Check sheet for the modelled part. Datum: model origin and axes. Units: mm. A direction names the side the tool comes from. Coordinates: 2 decimals unless noted, no trailing zeros. Loops run counter-clockwise (first coordinate to the right, second up) from the corner with the lowest first, then second, coordinate; pieces in that order, holes last. Notation, with made-up numbers: M -19,27.5 L 14,27.5 A21 ccw 14,34.5 Z; hole C 85.5,-26 d1. An arc over 180 degrees is marked long. Answer in a Markdown table with one row per item. Add a question column.
```python
from build123d import *

# Parameters (mm, degrees)
SKETCH_1_W          = 80
SKETCH_1_H          = 28
SKETCH_1_R          = 4.25
SKETCH_1_R_2        = 2
EXTRUDE_1_DEPTH     = 3
FILLET_2_RADIUS     = 14
FILLET_2_LENGTH     = 3
EXTRUDE_3_DEPTH     = 3
SKETCH_5_W          = 18.5
SKETCH_5_H          = 18.5
EXTRUDE_4_DEPTH     = 3
FILLET_3_R          = 18.5
EXTRUDE_5_DEPTH     = 3
CUT_EXTRUDE_1_REACH = 70.323
SKETCH_10_R         = 1.75


with BuildPart() as part:
    # 草图1 → 凸台-拉伸1 (new body)
    with BuildSketch(Plane(origin=(0, 0, 0), x_dir=(1, 0, 0), z_dir=(0, 1, 0))):
        Rectangle(SKETCH_1_W, SKETCH_1_H)
        with Locations(Location((25, 0, 0), (0, 0, 270))):
            Circle(SKETCH_1_R, mode=Mode.SUBTRACT)
        with Locations(Location((-25, 0, 0), (0, 0, 270))):
            Circle(SKETCH_1_R_2, mode=Mode.SUBTRACT)
    extrude(amount=EXTRUDE_1_DEPTH)

    # 圆角2: full round fillet: the end face becomes a half cylinder, R = half its width
    fillet_2_face = Plane((40, 1.5, 0), x_dir=(0, -1, 0), z_dir=(1, 0, 0))  # on the end face: x along it, z out of the body
    fillet_2_slab = fillet_2_face.offset(-FILLET_2_RADIUS / 2) * Box(FILLET_2_LENGTH, 2 * FILLET_2_RADIUS, FILLET_2_RADIUS, mode=Mode.PRIVATE)  # the body's end, R deep
    fillet_2_round = Plane((26, 1.5, 0), x_dir=(1, 0, 0), z_dir=(0, -1, 0)) * Cylinder(FILLET_2_RADIUS, FILLET_2_LENGTH, mode=Mode.PRIVATE)  # its axis R under the face
    add(fillet_2_slab - fillet_2_round, mode=Mode.SUBTRACT)

    # 草图4 → 凸台-拉伸3 (add)
    with BuildSketch(Plane.XZ):
        with BuildLine():
            Line((-40, 14), (-40, -14))
            ThreePointArc((-40, -14), (-54, 0), (-40, 14))
        make_face()
    extrude(amount=-EXTRUDE_3_DEPTH)

    # 草图5 → 凸台-拉伸4 (add)
    with BuildSketch(Plane(origin=(0, 0, 0), x_dir=(-1, 0, 0), z_dir=(0, -1, 0))):
        with Locations((12.25, -23.25)):
            Rectangle(SKETCH_5_W, SKETCH_5_H)
    extrude(amount=-EXTRUDE_4_DEPTH)

    # 圆角3
    fillet_3_edges = [part.edges().sort_by_distance(p)[0] for p in [
        (-21.5, 1.5, 14),
        (-3, 1.5, 14),
    ]]
    fillet(fillet_3_edges, radius=FILLET_3_R - 0.0001)  # a hair under: the kernel refuses the full size

    # 草图6 → 凸台-拉伸5 (add)
    with BuildSketch(Plane.XZ):
        with BuildLine():
            Line((-21.5, 32.5), (-3, 32.5))
            ThreePointArc((-3, 32.5), (-12.25, 41.75), (-21.5, 32.5))
        make_face()
    extrude(amount=-EXTRUDE_5_DEPTH)

    # 草图10 → 切除-拉伸1 (cut, up to next)
    with BuildSketch(Plane.XZ, mode=Mode.PRIVATE) as cut_extrude_1_sk1:
        with Locations(Location((-12.25, 37.5, 0), (0, 0, 270))):
            Circle(SKETCH_10_R)
    cut_extrude_1_tool1 = extrude(cut_extrude_1_sk1.sketch, amount=-CUT_EXTRUDE_1_REACH, mode=Mode.PRIVATE) & part.part
    # 草图10 → 切除-拉伸1 (cut, up to next)
    with BuildSketch(Plane.XZ, mode=Mode.PRIVATE) as cut_extrude_1_sk2:
        with Locations(Location((-7.919872981, 30, 0), (0, 0, 270))):
            Circle(SKETCH_10_R)
    cut_extrude_1_tool2 = extrude(cut_extrude_1_sk2.sketch, amount=-CUT_EXTRUDE_1_REACH, mode=Mode.PRIVATE) & part.part
    # 草图10 → 切除-拉伸1 (cut, up to next)
    with BuildSketch(Plane.XZ, mode=Mode.PRIVATE) as cut_extrude_1_sk3:
        with Locations(Location((-16.580127019, 30, 0), (0, 0, 270))):
            Circle(SKETCH_10_R)
    cut_extrude_1_tool3 = extrude(cut_extrude_1_sk3.sketch, amount=-CUT_EXTRUDE_1_REACH, mode=Mode.PRIVATE) & part.part
    # 草图10 → 切除-拉伸1 (cut, up to next)
    with BuildSketch(Plane.XZ, mode=Mode.PRIVATE) as cut_extrude_1_sk4:
        with Locations(Location((-18.244078093, 21.233684631, 0), (0, 0, 270))):
            Circle(SKETCH_10_R)
    cut_extrude_1_tool4 = extrude(cut_extrude_1_sk4.sketch, amount=-CUT_EXTRUDE_1_REACH, mode=Mode.PRIVATE) & part.part
    # 草图10 → 切除-拉伸1 (cut, up to next)
    with BuildSketch(Plane.XZ, mode=Mode.PRIVATE) as cut_extrude_1_sk5:
        with Locations(Location((-2.240350538, 12.7860315, 0), (0, 0, 270))):
            Circle(SKETCH_10_R)
    cut_extrude_1_tool5 = extrude(cut_extrude_1_sk5.sketch, amount=-CUT_EXTRUDE_1_REACH, mode=Mode.PRIVATE) & part.part
    add(cut_extrude_1_tool1.solids().sort_by_distance((-12.25, 0, 37.5))[0], mode=Mode.SUBTRACT)
    add(cut_extrude_1_tool2.solids().sort_by_distance((-7.919873, 0, 30))[0], mode=Mode.SUBTRACT)
    add(cut_extrude_1_tool3.solids().sort_by_distance((-16.580127, 0, 30))[0], mode=Mode.SUBTRACT)
    add(cut_extrude_1_tool4.solids().sort_by_distance((-18.244078, 0, 21.233685))[0], mode=Mode.SUBTRACT)
    add(cut_extrude_1_tool5.solids().sort_by_distance((-2.240351, 0, 12.786031))[0], mode=Mode.SUBTRACT)


solid = part.part
```
Q1. Cross-section at B-B (z = 30). Record the cut outline in (x, y), plus the area to 3 significant figures.
Q2. Mould release check, pull along X, two halves, no side actions. Record for faces 3 (the face through (-27.06, 1.52, 19.28)), 4 (the face through (29.214, 1.479, -0.553)), 5 (the face through (40, 1, 0)): released by +X, released by -X, zero draft, split by the parting line, or undercut.
Q3. Thickness scan on L1, parallel to X at y = 0.7, z = 0; L2, parallel to X at y = 2, z = 30; L3, parallel to Z at x = -40, y = 2. Record the ranges inside material, lowest first.
Q4. Cross-section at C-C (z = 37.5). Record the cut outline in (x, y).
Q5. Cross-section at A-A (x = 25). Record the cut outline in (y, z), plus the area to 3 significant figures.
Q6. Access from +Z, -Z, +X, -X, +Y, -Y to the whole of each face (thin tool, end or side, straight path). Record for faces 1 (the face through (21, 1, 14)), 2 (the face through (-12.047, 1.479, 41.748)).
Q7. Cross-section at D-D (y = 2.4). Count the separate pieces of the cut face and the enclosed holes in it, plus the area to 3 significant figures.
Q8. Go/stop test with flat-tipped pins: pin 1 (3 mm diameter, centred on x = -7.92, z = 30, fed in from -Y); pin 2 (0.9 mm diameter, centred on x = 21, y = 2, fed in from +Z); pin 3 (1.5 mm diameter, centred on x = -44, y = 2.5, fed in from -Z). Record where each tip stops, or that it passes through.
Answer key:
| question | item | result |
|---|---|---|
| 1 | outline | M -21.67,0 L -18.33,0 L -18.33,3 L -21.67,3 Z; M -14.83,0 L -9.67,0 L -9.67,3 L -14.83,3 Z; M -6.17,0 L -2.83,0 L -2.83,3 L -6.17,3 Z |
| 1 | area | 35.5 mm^2 |
| 2 | face 3 | released by -X |
| 2 | face 4 | undercut |
| 2 | face 5 | released by +X |
| 3 | L1 | -54 to -27, -23 to 20.75, 29.25 to 40 |
| 3 | L2 | -21.67 to -18.33, -14.83 to -9.67, -6.17 to -2.83 |
| 3 | L3 | -14 to 14 |
| 4 | outline | M -20.03,0 L -14,0 L -14,3 L -20.03,3 Z; M -10.5,0 L -4.47,0 L -4.47,3 L -10.5,3 Z |
| 5 | outline | M 0,-14 L 3,-14 L 3,-4.25 L 0,-4.25 Z; M 0,4.25 L 3,4.25 L 3,14 L 0,14 Z |
| 5 | area | 58.5 mm^2 |
| 6 | face 1 | +Z, +X, +Y, -Y |
| 6 | face 2 | +Z, +Y, -Y |
| 7 | separate pieces | 1 |
| 7 | enclosed holes | 7 |
| 7 | area | 2,970 mm^2 |
| 8 | pin 1 | through |
| 8 | pin 2 | z = 14 |
| 8 | pin 3 | z = -13.62 |
